Could you check a few things on this model? Use its own coordinates, in mm. Face numbers are marked on the shaded views. A direction names the side the tool comes from. Give positions to 0.01 mm unless a question says otherwise; leave off trailing zeros. Order: outer loops, then holes, each group sorted by start corner. A loop starts at its lowest first (then second) coordinate and runs counter-clockwise, first axis right, second up.
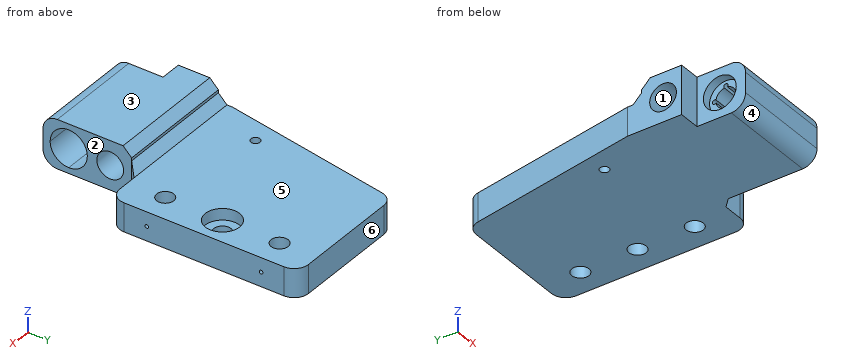
from build123d import *

# Parameters (mm, degrees)
SKETCH1_R             = 6
BOSS_EXTRUDE1_DEPTH   = 34
SKETCH2_W             = 115
SKETCH2_H             = 138
CUT_EXTRUDE1_DEPTH    = 14
SKETCH3_R             = 12
CUT_EXTRUDE2_DEPTH    = 8
SKETCH4_R             = 6
CUT_EXTRUDE3_DEPTH    = 225.686448189
FILLET1_R             = 10
CHAMFER1_SIZE         = 6
CUT_EXTRUDE8_DEPTH    = 34
SKETCH11_R            = 11.5
CUT_EXTRUDE9_DEPTH    = 6
SKETCH12_R            = 7
CUT_EXTRUDE10_DEPTH   = 224.588908491
FILLET3_R             = 10
SKETCH13_R            = 1.5
CUT_EXTRUDE11_DEPTH   = 224.588908491
M3_TAPPED_HOLE1_D     = 2.5
M3_TAPPED_HOLE1_DEPTH = 20
M3_TAPPED_HOLE1_TIP   = 0.751075774
SKETCH17_R            = 9.349207245
CUT_EXTRUDE12_DEPTH   = 234.197341372
SKETCH18_R            = 3.175
CUT_EXTRUDE13_DEPTH   = 20


with BuildPart() as part:
    # Sketch1 → Boss-Extrude1 (new body)
    with BuildSketch(Plane.XY):
        Polygon((0, 0), (70, 0), (70, 62), (76, 68), (100, 68), (100, 200), (7.876898591, 200), (-15, 72), (-15, 34), (0, 34), align=None)
        with Locations((81.891070834, 174)):
            Circle(SKETCH1_R, mode=Mode.SUBTRACT)
        with Locations((81.891070834, 94)):
            Circle(SKETCH1_R, mode=Mode.SUBTRACT)
    extrude(amount=BOSS_EXTRUDE1_DEPTH)

    # Sketch2 → Cut-Extrude1 (cut)
    with BuildSketch(Plane.XY.offset(34)):
        with Locations((42.5, 131)):
            Rectangle(SKETCH2_W, SKETCH2_H)
    extrude(amount=-CUT_EXTRUDE1_DEPTH, mode=Mode.SUBTRACT)

    # Sketch3 → Cut-Extrude2 (cut)
    with BuildSketch(Plane.XY.offset(20)):
        with Locations((81.891070834, 134)):
            Circle(SKETCH3_R)
    extrude(amount=-CUT_EXTRUDE2_DEPTH, mode=Mode.SUBTRACT)

    # Sketch4 → Cut-Extrude3 (cut, through all)
    with BuildSketch(Plane.XY.offset(12)):
        with Locations((81.891070834, 134)):
            Circle(SKETCH4_R)
    extrude(amount=-CUT_EXTRUDE3_DEPTH, mode=Mode.SUBTRACT)

    # Fillet1
    fillet1_edges = [part.edges().sort_by_distance(p)[0] for p in [
        (7.876898591, 200, 10),
        (100, 200, 10),
        (100, 68, 10),
    ]]
    fillet(fillet1_edges, radius=FILLET1_R)

    # Chamfer1
    chamfer1_edges = [part.edges().sort_by_distance(p)[0] for p in [
        (27.5, 62, 34),
        (27.5, 62, 20),
    ]]
    chamfer(chamfer1_edges, length=CHAMFER1_SIZE)

    # Sketch6 → Cut-Extrude8 (cut)
    with BuildSketch(Plane(origin=(70, 0, 0), x_dir=(0, 0, -1), z_dir=(1, 0, 0))):
        with BuildLine():
            ThreePointArc((-17, 31), (-30, 18), (-17, 5))
            Line((-17, 5), (-17, 31))
        make_face()
        with BuildLine():
            Line((-17, 31), (-17, 5))
            ThreePointArc((-17, 5), (-7.807611845, 8.807611845), (-4, 18))
            ThreePointArc((-4, 18), (-7.807611845, 27.192388155), (-17, 31))
        make_face()
    extrude(amount=-CUT_EXTRUDE8_DEPTH, mode=Mode.SUBTRACT)

    # Sketch11 → Cut-Extrude9 (cut)
    with BuildSketch(Plane.ZY):
        with Locations(Location((17, 18, 0), (0, 0, 270))):
            Circle(SKETCH11_R)
    extrude(amount=-CUT_EXTRUDE9_DEPTH, mode=Mode.SUBTRACT)

    # Sketch12 → Cut-Extrude10 (cut, through all)
    with BuildSketch(Plane.ZY.offset(-6)):
        with Locations(Location((17, 18, 0), (0, 0, 270))):
            Circle(SKETCH12_R)
    extrude(amount=-CUT_EXTRUDE10_DEPTH, mode=Mode.SUBTRACT)

    # Fillet3
    fillet3_edges = [part.edges().sort_by_distance(p)[0] for p in [
        (35, 0, 0),
        (35, 0, 34),
    ]]
    fillet(fillet3_edges, radius=FILLET3_R)

    # Sketch13 → Cut-Extrude11 (cut, through all)
    with BuildSketch(Plane.ZY.offset(-6)):
        with Locations((17, 26)):
            Circle(SKETCH13_R)
        with Locations((25, 18)):
            Circle(SKETCH13_R)
        with Locations((17, 10)):
            Circle(SKETCH13_R)
        with Locations((9, 18)):
            Circle(SKETCH13_R)
    extrude(amount=-CUT_EXTRUDE11_DEPTH, mode=Mode.SUBTRACT)

    # M3 Tapped Hole1
    with Locations(Plane(origin=(100, 0, 0), x_dir=(0, 0, -1), z_dir=(1, 0, 0))):
        with Locations((-10, 174), (-10, 94)):
            Hole(M3_TAPPED_HOLE1_D / 2, depth=M3_TAPPED_HOLE1_DEPTH)
            with Locations((0, 0, -(M3_TAPPED_HOLE1_DEPTH + M3_TAPPED_HOLE1_TIP / 2))):  # 118° drill point
                Cone(0, M3_TAPPED_HOLE1_D / 2, M3_TAPPED_HOLE1_TIP, mode=Mode.SUBTRACT)

    # Sketch17 → Cut-Extrude12 (cut, through all)
    with BuildSketch(Plane.ZY.offset(15)):
        with Locations(Location((17, 47, 0), (0, 0, 270))):
            Circle(SKETCH17_R)
    extrude(amount=-CUT_EXTRUDE12_DEPTH, mode=Mode.SUBTRACT)

    # Sketch18 → Cut-Extrude13 (cut)
    with BuildSketch(Plane(origin=(0, 0, 0), x_dir=(-1, 0, 0), z_dir=(0, 0, -1))):
        with Locations((-5, 102.220957779)):
            Circle(SKETCH18_R)
    extrude(amount=-CUT_EXTRUDE13_DEPTH, mode=Mode.SUBTRACT)


solid = part.part
Item 1: Imagine slicing it at B-B on y = 134. List the corners of the cut face in (x, z) for me.
Findings:
outline: (-3.92, 0) - (75.89, 0) - (75.89, 12) - (69.89, 12) - (69.89, 20) - (-3.92, 20) - close; (87.89, 0) - (100, 0) - (100, 20) - (93.89, 20) - (93.89, 12) - (87.89, 12) - close
Item 2: Imagine slicing it at C-C on x = 51. List the corners of the cut face in (y, z) for me.
Findings:
outline: (0, 10) arc R10 ccw to (10, 0) - (200, 0) - (200, 20) - (68, 20) - (62, 26) - (62, 28) - (56, 34) - (10, 34) arc R10 ccw to (0, 24) - close; hole circle Ø26 at (18, 17); hole circle Ø18.7 at (47, 17)
Item 3: For the marked faces 5 and 6, which set-ups out of +Z, -Z, +X, -X, +Y, -Y let a thin tool reach every point of the face, with its end or its side?
Findings:
face 5: +Z, +X, -X, +Y
face 6: +Z, -Z, +X, -X, +Y
Item 4: Imagine slicing it at D-D on z = 32. List the corners of the cut face in (x, y) for me.
Findings:
outline: (-15, 34) - (0, 34) - (0, 4) - (70, 4) - (70, 58) - (-15, 58) - close
Item 5: For pin 1 (3 mm diameter, centred on y = 94, z = 10, fed in from -X); pin 2 (7 mm diameter, centred on x = 81, z = 12.5, fed in from -Y); pin 3 (11 mm diameter, centred on x = 81.89, y = 94, fed in from -Z); pin 4 (14.5 mm diameter, centred on x = 81.89, y = 134, fed in from +Z), each with a flat end and sliding along its axis, tell me the tip position at first contact or that it passes through.
Findings:
pin 1: stops at x = -11.34
pin 2: stops at y = 68
pin 3: passes through
pin 4: stops at z = 12
Item 6: Imagine slicing it at A-A on x = 31. List the corners of the cut face in (y, z) for me.
Findings:
outline: (0, 10) arc R10 ccw to (10, 0) - (200, 0) - (200, 20) - (68, 20) - (62, 26) - (62, 28) - (56, 34) - (10, 34) arc R10 ccw to (0, 24) - close; hole (11.08, 15.96) arc R7 ccw to (16.96, 10.08) arc R1.5 ccw (long way) to (19.04, 10.08) arc R7 ccw to (24.92, 15.96) arc R1.5 ccw (long way) to (24.92, 18.04) arc R7 ccw to (19.04, 23.92) arc R1.5 ccw (long way) to (16.96, 23.92) arc R7 ccw to (11.08, 18.04) arc R1.5 ccw (long way) to start; hole circle Ø18.7 at (47, 17)
Item 7: Please list where these lines run through material, in increasing order: line 1 along Z through (x, y) = (56.5, 18.5); line 2 along Y through (x, z) = (86.5, 9); line 3 along Z through (x, y) = (91, 94).
Findings:
line 1: z = 0 to 4.01, 29.99 to 34
line 2: y = 68 to 90.16, 97.84 to 130.16, 137.84 to 170.16, 177.84 to 200
line 3: z = 0 to 8.75, 11.25 to 20
Item 8: We'd pull the mould along Z, two halves only. Please class the marked faces 1, 2, 3 and 4: +Z half, -Z half, draft (parallel to the pull), parting line (faces both ways), or undercut.
Findings:
face 1: undercut
face 2: draft
face 3: +Z half
face 4: -Z half
